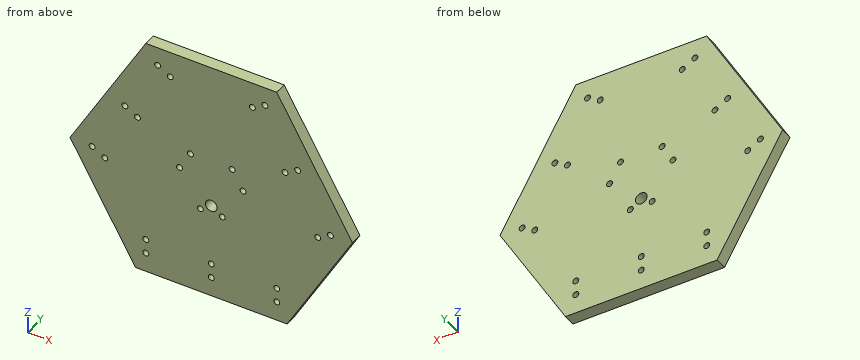
from build123d import *

# Parameters (mm, degrees)
BOSS_EXTRUDE1_DEPTH = 10
SKETCH2_OUTSIDE_W   = 431.978
SKETCH2_OUTSIDE_H   = 386.427
CUT_EXTRUDE1_DEPTH  = 10
SKETCH3_R           = 4.800665827
CUT_EXTRUDE2_DEPTH  = 10
SKETCH4_R           = 2.45
CUT_EXTRUDE3_DEPTH  = 10
SKETCH5_R           = 2.45
CUT_EXTRUDE4_DEPTH  = 10


with BuildPart() as part:
    # Sketch1 → Boss-Extrude1 (new body)
    with BuildSketch(Plane(origin=(0, 0, 0), x_dir=(1, 0, 0), z_dir=(0, 1, 0))):
        Polygon((170, 98.149545762), (-170, 98.149545762), (0, -196.299091524), align=None)
    extrude(amount=BOSS_EXTRUDE1_DEPTH)

    # Sketch2 outside → Cut-Extrude1 (cut)
    with BuildSketch(Plane(origin=(0, 10, 0), x_dir=(1, 0, 0), z_dir=(0, 1, 0))):
        with Locations((0, -49.0745)):
            Rectangle(SKETCH2_OUTSIDE_W, SKETCH2_OUTSIDE_H)
        Polygon((178.5, -103.05702305), (0, 206.114046101), (-178.5, -103.05702305), align=None, mode=Mode.SUBTRACT)
    extrude(amount=-CUT_EXTRUDE1_DEPTH, mode=Mode.SUBTRACT)

    # Sketch3 → Cut-Extrude2 (cut)
    with BuildSketch(Plane(origin=(0, 10, 0), x_dir=(1, 0, 0), z_dir=(0, 1, 0))):
        with Locations(Location((0, 18.713723456, 0), (0, 0, 270))):
            Circle(SKETCH3_R)
    extrude(amount=-CUT_EXTRUDE2_DEPTH, mode=Mode.SUBTRACT)

    # Sketch4 → Cut-Extrude3 (cut)
    with BuildSketch(Plane(origin=(0, 10, 0), x_dir=(1, 0, 0), z_dir=(0, 1, 0))):
        with Locations(Location((0, 82.049545762, 0), (0, 0, 270))):
            Circle(SKETCH4_R)
        with Locations(Location((-53.840790268, 82.049545762, 0), (0, 0, 270))):
            Circle(SKETCH4_R)
        with Locations(Location((-53.840790268, 70.049545762, 0), (0, 0, 270))):
            Circle(SKETCH4_R)
        with Locations(Location((0, 70.049545762, 0), (0, 0, 270))):
            Circle(SKETCH4_R)
        with Locations(Location((71.056990999, -41.024772881, 0), (0, 0, 270))):
            Circle(SKETCH4_R)
        with Locations(Location((60.664686154, -35.024772881, 0), (0, 0, 270))):
            Circle(SKETCH4_R)
        with Locations(Location((-71.056990999, -41.024772881, 0), (0, 0, 270))):
            Circle(SKETCH4_R)
        with Locations(Location((-60.664686154, -35.024772881, 0), (0, 0, 270))):
            Circle(SKETCH4_R)
        with Locations(Location((-87.585081287, 11.60271925, 0), (0, 0, 270))):
            Circle(SKETCH4_R)
        with Locations(Location((-97.977386133, 5.60271925, 0), (0, 0, 270))):
            Circle(SKETCH4_R)
        with Locations(Location((53.840790268, 82.049545762, 0), (0, 0, 270))):
            Circle(SKETCH4_R)
        with Locations(Location((53.840790268, 70.049545762, 0), (0, 0, 270))):
            Circle(SKETCH4_R)
        with Locations(Location((97.977386133, 5.60271925, 0), (0, 0, 270))):
            Circle(SKETCH4_R)
        with Locations(Location((87.585081287, 11.60271925, 0), (0, 0, 270))):
            Circle(SKETCH4_R)
        with Locations(Location((44.136595865, -87.652265013, 0), (0, 0, 270))):
            Circle(SKETCH4_R)
        with Locations(Location((33.74429102, -81.652265013, 0), (0, 0, 270))):
            Circle(SKETCH4_R)
        with Locations(Location((-33.74429102, -81.652265013, 0), (0, 0, 270))):
            Circle(SKETCH4_R)
        with Locations(Location((-44.136595865, -87.652265013, 0), (0, 0, 270))):
            Circle(SKETCH4_R)
    extrude(amount=-CUT_EXTRUDE3_DEPTH, mode=Mode.SUBTRACT)

    # Sketch5 → Cut-Extrude4 (cut)
    with BuildSketch(Plane(origin=(0, 10, 0), x_dir=(1, 0, 0), z_dir=(0, 1, 0))):
        with Locations(Location((26.106940443, -4.680544247, 0), (0, 0, 270))):
            Circle(SKETCH5_R)
        with Locations(Location((17.106940443, -20.269001515, 0), (0, 0, 270))):
            Circle(SKETCH5_R)
        with Locations(Location((-17.106940443, -20.269001515, 0), (0, 0, 270))):
            Circle(SKETCH5_R)
        with Locations(Location((-26.106940443, -4.680544247, 0), (0, 0, 270))):
            Circle(SKETCH5_R)
        with Locations(Location((-9, 24.949545762, 0), (0, 0, 270))):
            Circle(SKETCH5_R)
        with Locations(Location((9, 24.949545762, 0), (0, 0, 270))):
            Circle(SKETCH5_R)
    extrude(amount=-CUT_EXTRUDE4_DEPTH, mode=Mode.SUBTRACT)


solid = part.part
Can you work these out from the model? Positions are in its coordinate system, mm. Round coordinates to 2 decimals unless told otherwise and drop trailing zeros. Write each loop counter-clockwise with the first axis right and the second up, starting at its lowest first coordinate (ties: lowest second). Pieces come first, ordered by that corner, then holes. Notation, with made-up numbers: (51, 89.5) - (99, 89.5) arc R14 cw to (99, 100.5) - close; hole circle Ø2 at (3.5, 1). An arc over 180 degrees is marked (long way). Write each question's results on one line, items separated by ' | '. Start each with the question number.
1) For pin 1 Ø4 at (x, y) = (84, 5) entering from +Z; pin 2 Ø3 at (x, z) = (-71.06, 41.02) entering from -Y; pin 3 Ø1 at (y, z) = (4, 23) entering from +X; pin 4 Ø2 at (y, z) = (1, -39) entering from -X, each with a flat end and sliding along its axis, tell me the tip position at first contact or that it passes through.
2) Suppose I cut it at C-C (x = 82). List the corners of the cut face in (y, z) for me, and give its area (3 significant figures).
3) Please list where these lines run through material, in increasing order: line 1 (Z direction, x = 17, y = 2.5); line 2 (X direction, y = 5.5, z = 79.5); line 3 (X direction, y = 6.75, z = 35).
4) Suppose I cut it at A-A (y = 4.5). Give the number of separate pieces and of enclosed holes in the cut face, and give its area (3 significant figures).
5) Suppose I cut it at B-B (z = 59.5). List the corners of the cut face in (x, y) for me.
Here are the results:
1) pin 1: stops at z = 54.27 | pin 2: passes through | pin 3: stops at x = 100.34 | pin 4: stops at x = -97.06
2) outline: (0, -64.09) - (10, -64.09) - (10, 54.27) - (0, 54.27) - close | area: 1,180 mm2
3) line 1: z = -98.15 to 17.82, 22.72 to 103.06 | line 2: x = -67.43 to -34.91, -32.57 to 32.57, 34.91 to 67.43 | line 3: x = -93.13 to -63.11, -58.21 to 58.21, 63.11 to 93.13
4) separate pieces: 1 | enclosed holes: 25 | area: 34,500 mm2
5) outline: (-78.98, 0) - (78.98, 0) - (78.98, 10) - (-78.98, 10) - close
